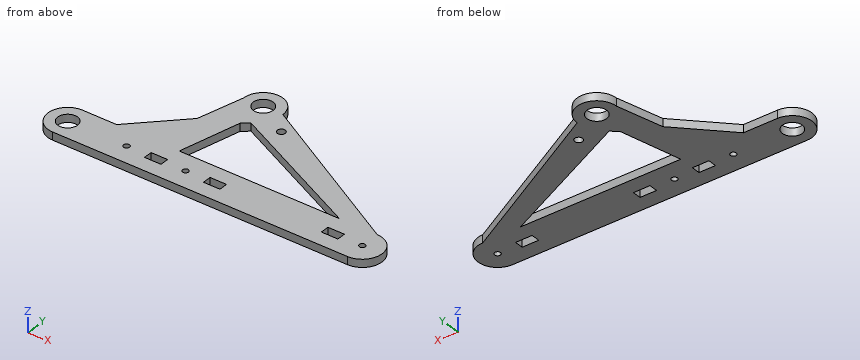
from build123d import *

# Parameters (mm, degrees)
SKETCH_1_R      = 5.03
SKETCH_1_R_2    = 5.04
SKETCH_1_R_3    = 1.5
SKETCH_1_R_4    = 2
SKETCH_1_W      = 8.4
SKETCH_1_H      = 4.4
EXTRUDE_1_DEPTH = 4
EXTRUDE_2_DEPTH = 4


with BuildPart() as part:
    # 草图1 → 凸台-拉伸1 (new body)
    with BuildSketch(Plane.XY):
        with BuildLine():
            Line((0, 10), (34.696699141, 10))
            Line((34.696699141, 10), (46.568305139, 56.568542495))
            ThreePointArc((46.568305139, 56.568542495), (56.568542495, 66.568779851), (66.568779851, 56.568542495))
            Line((66.568779851, 56.568542495), (150, 10))
            ThreePointArc((150, 10), (160, 0), (150, -10))
            Line((150, -10), (0, -10))
            ThreePointArc((0, -10), (-10, 0), (0, 10))
        make_face()
        Circle(SKETCH_1_R, mode=Mode.SUBTRACT)
        with Locations((56.568542495, 56.568542495)):
            Circle(SKETCH_1_R_2, mode=Mode.SUBTRACT)
        with Locations((30, 0)):
            Circle(SKETCH_1_R_3, mode=Mode.SUBTRACT)
        with Locations((60, 0)):
            Circle(SKETCH_1_R_3, mode=Mode.SUBTRACT)
        with Locations((150, 0)):
            Circle(SKETCH_1_R_3, mode=Mode.SUBTRACT)
        with Locations((73.677090033, 46.210086957)):
            Circle(SKETCH_1_R_4, mode=Mode.SUBTRACT)
        with Locations((75, 0)):
            Rectangle(SKETCH_1_W, SKETCH_1_H, mode=Mode.SUBTRACT)
        with Locations((45, 0)):
            Rectangle(SKETCH_1_W, SKETCH_1_H, mode=Mode.SUBTRACT)
        with Locations((135, 0)):
            Rectangle(SKETCH_1_W, SKETCH_1_H, mode=Mode.SUBTRACT)
        Polygon((56.568542495, 40.992584384), (49.2, 10), (130.8, 10), (60, 43.844151412), align=None, mode=Mode.SUBTRACT)
    extrude(amount=EXTRUDE_1_DEPTH)

    # 草图2 → 凸台-拉伸2 (add)
    with BuildSketch(Plane.XY.offset(4)):
        Polygon((34.696699141, 10), (40.63250214, 33.284271247), (17.348349571, 10), align=None)
    extrude(amount=-EXTRUDE_2_DEPTH)


solid = part.part
Can you work these out from the model? Positions are in its coordinate system, mm. Give positions to 0.01 mm unless a question says otherwise; leave off trailing zeros. Order: outer loops, then holes, each group sorted by start corner. A loop starts at its lowest first (then second) coordinate and runs counter-clockwise, first axis right, second up. Notation, with made-up numbers: M 58.25,43.25 L 112.25,43.25 A18 cw 112.25,75.25 Z; hole C 77.5,42 d4. An arc over 180 degrees is marked long. Use one line per item in the form item = value.
Item 1: If I drill on line 1 along Y through (x, z) = (58, 0.5); line 2 along Y through (x, z) = (30, 2.45); line 3 along Y through (x, z) = (104, 3.5), over which ranges is the centre line in solid material (lowest first)? Write a range as [from, to].
Values follow:
line_1 = [-10, 10], [42.18, 51.74], [61.4, 66.47]
line_2 = [-10, -1.5], [1.5, 22.65]
line_3 = [-10, 10], [22.81, 35.68]
Item 2: If we section it at B-B, the plane y = 55: Write out the boundary of the cut face in (x, z), and give its area (3 significant figures).
Values follow:
outline = M 46.17,0 L 51.78,0 L 51.78,4 L 46.17,4 Z; M 61.36,0 L 69.38,0 L 69.38,4 L 61.36,4 Z
area = 54.5 mm^2
Item 3: If we section it at D-D, the plane x = 8: Write out the boundary of the cut face in (y, z), and give its area (3 significant figures).
Values follow:
outline = M -10,0 L 10,0 L 10,4 L -10,4 Z
area = 80.0 mm^2
Item 4: If we section it at A-A, the plane x = 30: Write out the boundary of the cut face in (y, z).
Values follow:
outline = M -10,0 L -1.5,0 L -1.5,4 L -10,4 Z; M 1.5,0 L 22.65,0 L 22.65,4 L 1.5,4 Z
Item 5: Will these pins go through, and if not, where does the flat tip stop? pin 1 Ø1 at (y, z) = (30.5, 2) entering from -X; pin 2 Ø16 at (x, y) = (0, 0) entering from +Z; pin 3 Ø1.2 at (y, z) = (1, 2.5) entering from -X; pin 4 Ø1.8 at (x, y) = (150, 0) entering from -Z.
Values follow:
pin_1 = 37.35
pin_2 = 4
pin_3 = -9.99
pin_4 = through
Item 6: If we section it at C-C, the plane z = 3: Count the separate pieces of the cut face and the enclosed holes in it, and give its area (3 significant figures).
Values follow:
separate_pieces = 1
enclosed_holes = 10
area = 5,100 mm^2
